Autodesk Inventor part; units mm, degrees
ref_plane "YZ Plane" through (0, 0, 0) normal (1, 0, 0) x (0, 1, 0)
ref_plane "XZ Plane" through (0, 0, 0) normal (0, 1, 0) x (-1, 0, 0)
ref_plane "XY Plane" through (0, 0, 0) normal (0, 0, 1) x (1, 0, 0)
sketch "スケッチ8" plane through (0, 1.5, 0) normal (0, 1, 0) x (1, 0, 0)
  line L0 (-21.5, -23.5431) -> (-21.5, 0)
  line L1 (-21.5, -0.35) -> (-26.5, -0.35)
  line L2 (-26.5, -0.35) -> (-26.5, -3.35)
  line L3 (-26.5, -3.35) -> (-21.5, -3.35)
  line L4 (-21.5, -3.35) -> (-21.5, -0.35)
  line L5 (21.5, 0) -> (21.5, -23.5431)
  line L6 (21.5, -0.35) -> (26.5, -0.35)
  line L7 (26.5, -0.35) -> (26.5, -3.35)
  line L8 (26.5, -3.35) -> (21.5, -3.35)
  line L9 (21.5, -3.35) -> (21.5, -0.35)
  line L10 (-21.5, 0) -> (-14, 0)
  point P0 (0, 0)
  point P1 (-26.5, -1.85)
  dimension "d28" = 5
  dimension "d29" = 3
  dimension "d30" = 1.85
sketch "スケッチ1" plane through (0, 0, 0) normal (0, 1, 0) x (-1, 0, 0)
  line L0 (21.5, 0) -> (-21.5, 0)
  line L1 (-21.5, 0) -> (-21.5, 25.1)
  line L2 (-21.5, 25.1) -> (21.5, 25.1)
  line L3 (21.5, 25.1) -> (21.5, 0)
  point P0 (0, 0)
  point P1 (0, 0)
  dimension "d0" = 25.1
  dimension "d1" = 43
extrude "プレート1" add sketch "スケッチ1" along normal blind 1.5
sketch "スケッチ3" plane through (0, 1.5, 0) normal (0, 1, 0) x (1, 0, 0)
  line L0 (21.5, 0) -> (-21.5, 0)
  line L1 (-20, 0) -> (-20, -17.1)
  line L2 (20, 0) -> (20, -17.1)
  line L3 (-21.5, -25.1) -> (-21.5, 0)
  line L4 (21.5, 0) -> (21.5, -25.1)
  line L5 (-20, -17.1) -> (20, -17.1)
  line L6 (-20, 0) -> (-14, 0)
  line L7 (-14, 0) -> (-14, -10.2)
  line L8 (-14, -10.2) -> (-20, -10.2)
  line L9 (-20, -10.2) -> (-20, 0)
  line L10 (20, 0) -> (14, 0)
  line L11 (14, 0) -> (14, -10.2)
  line L12 (14, -10.2) -> (20, -10.2)
  line L13 (20, -10.2) -> (20, 0)
  line L14 (-20, -10.2) -> (-21.5, -10.2)
  line L15 (20, -10.2) -> (21.5, -10.2)
  line L16 (21.5, -25.1) -> (-21.5, -25.1)
  arc A0 (-14, -10.2) -> (14, -10.2) centre (0, 0.5529) ccw
  point P0 (0, 0)
  point P1 (20, -10.2)
  point P2 (14, 0)
  point P3 (-14, 0)
  dimension "d5" = 1.5
  dimension "d6" = 1.5
  dimension "d7" = 6
  dimension "d8" = 10.2
  dimension "d9" = 8
extrude "押し出し2" cut sketch "スケッチ3" against normal through all contours L11 A0 L7 L0
sketch "スケッチ4" plane through (-21.5, 0, 25.1) normal (-1, 0, 0) x (0, 0, 1)
  line L0 (-0.5569, 2.6) -> (-0.5569, 0)
  line L1 (0, 0) -> (-25.1, 0)
  line L2 (-25.1, 0) -> (0, 0)
  line L3 (0, 0) -> (0, 1.5)
  line L4 (0, 1.5) -> (-25.1, 1.5)
  line L5 (-25.1, 0) -> (-25.1, 1.5)
  point P0 (-14.9, 0)
  point P1 (0, 0)
  point P2 (-0.5569, 1.5)
extrude "押し出し3" cut sketch "スケッチ4" against normal through all contours L4 L3 L1 L0
sketch "スケッチ5" plane through (0, 1.5, 0) normal (0, 1, 0) x (1, 0, 0)
  circle A0 centre (0, -21.5431) radius 0.8
  circle A1 centre (-13, -21.5431) radius 0.8
  circle A2 centre (13, -21.5431) radius 0.8
  line L0 (-21.5, -24.5431) -> (-21.5, 0)
  line L1 (-21.5, -23.5431) -> (21.5, -23.5431)
  line L2 (21.5, -24.5431) -> (-21.5, -24.5431)
  line L3 (21.5, 0) -> (21.5, -24.5431)
  point P0 (0, 0)
  point P1 (-21.5, -10.2)
  point P2 (21.5, -10.2)
  dimension "d16" = 1
extrude "切り取り1" cut sketch "スケッチ5" against normal blind 1.5
sheet face with bend "面3" sketch "スケッチ8" thickness 1.5 toward (0, -1, 0) bend radius 1.5
bend "曲げ2"
equation "\"d6\" = d5"
equation "\"d14\" = Thickness"
equation "\"d2\" = Thickness"
equation "\"d31\" = BendRadius"
equation "\"d32\" = BendReliefWidth"
equation "\"d34\" = MinimumRemnant"
equation "\"d33\" = BendReliefDepth"
equation "\"d35\" = TransitionRadius"
equation "\"BendRadius\" = Thickness"
equation "\"BendReliefWidth\" = Thickness"
equation "\"BendReliefDepth\" = 0.5 * Thickness"
equation "\"CornerReliefSize\" = 4 * Thickness"
equation "\"MinimumRemnant\" = 2 * Thickness"
equation "\"TransitionRadius\" = BendRadius"
equation "\"JacobiRadiusSize\" = BendRadius"
equation "\"GapSize\" = Thickness"
properties part number "chest_cover_base" material "アルミニウム 6061"
Verification items for the finished model (mm, model axes). A direction names the side the tool comes from. Give positions to 0.01 mm unless a question says otherwise; leave off trailing zeros. Write each loop counter-clockwise with the first axis right and the second up, starting at its lowest first coordinate (ties: lowest second). Pieces come first, ordered by that corner, then holes. Notation, with made-up numbers: M -23,80 L 34,80 A18 cw 34,95 Z; hole C 35.5,-21.5 d4. An arc over 180 degrees is marked long. Use CSV: the item, a comma, the result in double quotes.
1) Cross-section at B-B (z = 4). Enter the section's corners in (x, y), plus the area to 3 significant figures.
Final values:
outline,"M -21.5,0 L -14,0 L -14,1.5 L -21.5,1.5 Z; M 14,0 L 21.5,0 L 21.5,1.5 L 14,1.5 Z"
area,"22.5 mm²"
2) Cross-section at D-D (x = -8). Enter the section's corners in (y, z).
Final values:
outline,"M 0,15.18 L 1.5,15.18 L 1.5,23.54 L 0,23.54 Z"
3) Cross-section at A-A (x = 0). Enter the section's corners in (y, z), plus the area to 3 significant figures.
Final values:
outline,"M 0,17.1 L 1.5,17.1 L 1.5,20.74 L 0,20.74 Z; M 0,22.34 L 1.5,22.34 L 1.5,23.54 L 0,23.54 Z"
area,"7.26 mm²"
4) Access from +Z, -Z, +X, -X, +Y, -Y to the whole of each face (thin tool, end or side, straight path). Record for faces 5 (the face through (-24, 1, 0.35)), 6 (the face through (-24, 1, 3.35)), 7 (the face through (24, 1, 0.35)).
Final values:
face 5,"-Z, -X, +Y, -Y"
face 6,"+Z, -X, +Y, -Y"
face 7,"-Z, +X, +Y, -Y"
5) Release check for a two-part mould opening along Z. For faces 1 (the face through (-12.631, 0.76, 22.253)), 2 (the face through (0, 0, 20)), 3 (the face through (0.43, 0.76, 20.87)), 4 (the face through (0, 1, 23.543)) record: released by +Z, released by -Z, zero draft, split by the parting line, or undercut.
Final values:
face 1,"undercut"
face 2,"zero draft"
face 3,"undercut"
face 4,"released by +Z"
6) Material ranges on line 1 along X through (y, z) = (0.8, 5.75); line 2 along Z through (x, y) = (0, 0.55); line 3 along X through (y, z) = (1, 21.75), recorded low to high.
Final values:
line 1,"-21.5 to -14, 14 to 21.5"
line 2,"17.1 to 20.74, 22.34 to 23.54"
line 3,"-21.5 to -13.77, -12.23 to -0.77, 0.77 to 12.23, 13.77 to 21.5"
7) Go/stop test with flat-tipped pins: pin 1 Ø1.4 at (x, z) = (-13, 21.54) entering from +Y; pin 2 Ø1.8 at (x, z) = (0, 21.54) entering from -Y; pin 3 Ø0.8 at (x, y) = (24.5, 1) entering from +Z. Record where each tip stops, or that it passes through.
Final values:
pin 1,"through"
pin 2,"y = 0"
pin 3,"z = 3.35"
8) Cross-section at C-C (y = 0.5). Enter the section's corners in (x, z), plus the area to 3 significant figures.
Final values:
outline,"M -26.5,0.35 L -21.5,0.35 L -21.5,0 L -14,0 L -14,10.2 A17.65 cw 14,10.2 L 14,0 L 21.5,0 L 21.5,0.35 L 26.5,0.35 L 26.5,3.35 L 21.5,3.35 L 21.5,23.54 L -21.5,23.54 L -21.5,3.35 L -26.5,3.35 Z; hole C -13,21.54 d1.6; hole C 0,21.54 d1.6; hole C 13,21.54 d1.6"
area,"616 mm²"
